The model under review builds one solid part; all positions refer to its coordinate system, in mm. A direction names the side the tool comes from. Round coordinates to 2 decimals unless told otherwise and drop trailing zeros. Order: outer loops, then holes, each group sorted by start corner. A loop starts at its lowest first (then second) coordinate and runs counter-clockwise, first axis right, second up.
```python
from build123d import *

# Parameters (mm, degrees)
F1_DEPTH = 25.4
F3_DEPTH = 25.4
F4_R     = 6.9752629403
F5_DEPTH = 25.4
F7_DEPTH = 25.4
F9_DEPTH = 25.4


with BuildPart() as f1:
    # F0 (on Front) → F1 (new body)
    with BuildSketch(Plane.XZ):
        with BuildLine():
            Line((0, 25.2437964082), (0, 0))
            Line((0, 0), (82.55, 0))
            Line((82.55, 0), (82.55, 12.7))
            Line((82.55, 12.7), (25.4, 12.7))
            Line((25.4, 12.7), (25.4, 25.4))
            ThreePointArc((25.4, 25.4), (21.338721964, 34.038721964), (12.7, 38.1))
            ThreePointArc((12.7, 38.1), (3.9765521081, 34.0165085715), (0, 25.2437964082))
        make_face()
    extrude(amount=F1_DEPTH)

    # F2 (on face) → F3 (cut)
    with BuildSketch(Plane.XY.offset(12.7)):
        with BuildLine():
            ThreePointArc((70.5987364054, 0), (78.1138192484, -4.9013082489), (82.55, -12.7))
            Line((82.55, -12.7), (82.55, 0))
            Line((82.55, 0), (70.5987364054, 0))
        make_face()
        with BuildLine():
            Line((82.55, -25.4), (82.55, -12.7))
            ThreePointArc((82.55, -12.7), (78.6112135374, -20.4997420186), (71.376748383, -25.4))
            Line((71.376748383, -25.4), (82.55, -25.4))
        make_face()
    extrude(amount=-F3_DEPTH, mode=Mode.SUBTRACT)

    # F4 (on face) → F5 (cut)
    with BuildSketch(Plane.XZ.offset(25.4)):
        with Locations((12.887516059, 26.3950787485)):
            Circle(F4_R)
    extrude(amount=-F5_DEPTH, mode=Mode.SUBTRACT)

    # F6 (on face) → F7 (cut)
    with BuildSketch(Plane.XY.offset(12.7)):
        with BuildLine():
            ThreePointArc((46.7944949583, -13.4114921093), (44.5635810438, -8.0266435433), (39.1781151252, -5.7972203415))
            ThreePointArc((39.1781151252, -5.7972203415), (31.5668924837, -13.2917465926), (38.938654761, -21.0219312446))
            Line((38.938654761, -21.0219312446), (39.4217910365, -21.0219312446))
            ThreePointArc((39.4217910365, -21.0219312446), (44.6490666759, -18.7094999177), (46.7944949583, -13.4114921093))
        make_face()
        with BuildLine():
            ThreePointArc((63.1514803528, -21.0219312446), (55.9492219457, -13.2618150882), (63.4506483721, -5.7905012482))
            Line((63.4506483721, -5.7905012482), (39.1781151252, -5.7972203415))
            ThreePointArc((39.1781151252, -5.7972203415), (44.5635810438, -8.0266435433), (46.7944949583, -13.4114921093))
            ThreePointArc((46.7944949583, -13.4114921093), (44.6490666759, -18.7094999177), (39.4217910365, -21.0219312446))
            Line((39.4217910365, -21.0219312446), (63.1514803528, -21.0219312446))
        make_face()
        with BuildLine():
            ThreePointArc((63.9878644586, -21.0219312446), (69.1050628574, -18.6510647038), (71.1915926641, -13.4114921093))
            ThreePointArc((71.1915926641, -13.4114921093), (68.9169369742, -7.9800622737), (63.4506483721, -5.7905012482))
            ThreePointArc((63.4506483721, -5.7905012482), (55.9492219457, -13.2618150882), (63.1514803528, -21.0219312446))
            Line((63.1514803528, -21.0219312446), (63.9878644586, -21.0219312446))
        make_face()
    extrude(amount=-F7_DEPTH, mode=Mode.SUBTRACT)

    # F8 (on face) → F9 (cut)
    with BuildSketch(Plane.XY.offset(12.7)):
        with BuildLine():
            ThreePointArc((70.5987364054, 0), (77.1764816954, -5.287668523), (81.6851109266, -12.4219823629))
            ThreePointArc((81.6851109266, -12.4219823629), (77.8552746278, -19.9629105497), (71.376748383, -25.4))
            ThreePointArc((71.376748383, -25.4), (78.6112135374, -20.4997420186), (82.55, -12.7))
            ThreePointArc((82.55, -12.7), (78.1138192484, -4.9013082489), (70.5987364054, 0))
        make_face()
    extrude(amount=-F9_DEPTH, mode=Mode.SUBTRACT)


solid = f1.part
```
(1) Consider section A-A (y = -18). Write out the cut boundary in (x, z).
Data:
outline: (0, 0) - (33.1, 0) - (33.1, 12.7) - (25.4, 12.7) - (25.4, 25.4) arc R14.08 ccw to (12.7, 38.1) arc R13.9 ccw to (0, 25.24) - close; (69.66, 0) - (79.24, 0) - (79.24, 12.7) - (69.66, 12.7) - close; hole circle Ø13.95 at (12.89, 26.4)
(2) For faces 4 (the flat face through (25.4, -13, 19)), 5 (the flat face through (31, -13, 0)), 6 (the flat face through (51, -21.022, 6)), list the 3-axis set-ups (+Z, -Z, +X, -X, +Y, -Y) from which the entire face can be reached by the end or side of a thin tool; tool diameter is ignored.
Data:
face 4: +Z, +X, +Y, -Y
face 5: -Z, +X, -X, +Y, -Y
face 6: +Z, -Z
(3) Draft analysis for pull direction Y (two halves, no side actions). For faces 1 (the cylindrical face through (7.352, -12.878, 22.151)), 2 (the cylindrical face through (31.57, -13.13, 6.44)), 3 (the cylindrical face through (77.1, -5.2, 6.4)), state which applies: pulls with the +Y half, pulls with the -Y half, needs draft (parallel to the pull), parting line crosses it, or undercut.
Data:
face 1: needs draft
face 2: undercut
face 3: pulls with the +Y half
(4) Consider section C-C (x = 45.5). Write out the cut boundary in (y, z).
Data:
outline: (-25.4, 0) - (-21.02, 0) - (-21.02, 12.7) - (-25.4, 12.7) - close; (-5.8, 0) - (0, 0) - (0, 12.7) - (-5.8, 12.7) - close
(5) To check wall thickness, follow probe 1 along Y at (x, z) = (50, 7.5); probe 2 along Z at (x, y) = (74, -14.75); probe 3 along X at (y, z) = (-13, 10). State the ranges of each line that lie inside material, in increasing order.
Data:
probe 1: y = -25.4 to -21.02, -5.79 to 0
probe 2: z = 0 to 12.7
probe 3: x = 0 to 31.58, 71.18 to 81.52
(6) Consider section B-B (z = 3.5). Write out the cut boundary in (x, y), and give its area (3 significant figures).
Data:
outline: (0, -25.4) - (71.38, -25.4) arc R21.15 ccw to (81.69, -12.42) arc R25.68 ccw to (70.6, 0) - (0, 0) - close; hole (38.94, -21.02) - (63.99, -21.02) arc R7.62 ccw to (63.45, -5.79) - (39.18, -5.8) arc R7.61 ccw to start
area: 1,420 mm2
(7) Insertion check: pin 1 (8 mm diameter, centred on x = 10.5, y = -9, fed in from -Z); pin 2 (4 mm diameter, centred on y = -16, z = 25, fed in from +X); pin 3 (3 mm diameter, centred on x = 40.5, y = -7, fed in from +Z). Each pin has a flat end and moves straight along its axis. Give the tip position at first contact, or say it passes through.
Data:
pin 1: stops at z = 0
pin 2: stops at x = 25.4
pin 3: stops at z = 12.7
(8) Consider section D-D (y = -14.5). Write out the cut boundary in (x, z).
Data:
outline: (0, 0) - (31.64, 0) - (31.64, 12.7) - (25.4, 12.7) - (25.4, 25.4) arc R14.08 ccw to (12.7, 38.1) arc R13.9 ccw to (0, 25.24) - close; (71.11, 0) - (81, 0) - (81, 12.7) - (71.11, 12.7) - close; hole circle Ø13.95 at (12.89, 26.4)
